```python
from build123d import *

# Parameters (mm, degrees)
F0_R     = 2.1
F1_DEPTH = 2
F2_R     = 4.1
F2_R_2   = 2.1
F3_DEPTH = 2.67
F4_W     = 1
F4_H     = 4.975
F4_W_2   = 3.1
F5_DEPTH = 5


with BuildPart() as f1:
    # F0 (on Top) → F1 (new body)
    with BuildSketch(Plane.XY):
        with BuildLine():
            Line((0, 15), (0, 0))
            Line((0, 0), (17, 0))
            ThreePointArc((17, 0), (24.5, 7.5), (17, 15))
            Line((17, 15), (0, 15))
        make_face()
        with Locations((17, 7.5)):
            Circle(F0_R, mode=Mode.SUBTRACT)
    extrude(amount=F1_DEPTH)

    # F2 (on face) → F3 (join)
    with BuildSketch(Plane.XY.offset(2)):
        with Locations((17, 7.5)):
            Circle(F2_R)
        with Locations((17, 7.5)):
            Circle(F2_R_2, mode=Mode.SUBTRACT)
    extrude(amount=F3_DEPTH)

    # F4 (on face) → F5 (join)
    with BuildSketch(Plane(origin=(0, 0, 0), x_dir=(1, 0, 0), z_dir=(0, 0, -1))):
        with Locations((3.3, -3.9125)):
            Rectangle(F4_W, F4_H)
        with Locations((7.45, -3.9125)):
            Rectangle(F4_W_2, F4_H)
        with BuildLine():
            ThreePointArc((22.529693, -6.05), (22.771721, -5.927264), (22.815711, -5.659483))
            ThreePointArc((22.815711, -5.659483), (21.102936, -2.986031), (18.278593, -1.535505))
            ThreePointArc((18.278593, -1.535505), (18.027117, -1.595534), (17.915711, -1.828841))
            Line((17.915711, -1.828841), (17.915711, -3.503567))
            ThreePointArc((17.915711, -3.503567), (19.695084, -4.410256), (20.835036, -6.05))
            Line((20.835036, -6.05), (22.529693, -6.05))
        make_face()
        with BuildLine():
            ThreePointArc((17.915711, -13.171159), (18.027117, -13.404466), (18.278593, -13.464495))
            ThreePointArc((18.278593, -13.464495), (21.102936, -12.013969), (22.815711, -9.340517))
            ThreePointArc((22.815711, -9.340517), (22.771721, -9.072736), (22.529693, -8.95))
            Line((22.529693, -8.95), (20.835036, -8.95))
            ThreePointArc((20.835036, -8.95), (19.695084, -10.589744), (17.915711, -11.496433))
            Line((17.915711, -11.496433), (17.915711, -13.171159))
        make_face()
        with Locations((3.3, -11.0875)):
            Rectangle(F4_W, F4_H)
        with Locations((7.45, -11.0875)):
            Rectangle(F4_W_2, F4_H)
    extrude(amount=F5_DEPTH)


solid = f1.part
```
Design review of the part built by this model. Coordinates are the model's own, in mm. A direction names the side the tool comes from. Give positions to 0.01 mm unless a question says otherwise; leave off trailing zeros. Loops run counter-clockwise (first coordinate to the right, second up) from the corner with the lowest first, then second, coordinate; pieces in that order, holes last. Notation, with made-up numbers: M 42,88.5 L 54,88.5 A16 cw 54,115.5 Z; hole C -34.5,59.5 d4. An arc over 180 degrees is marked long. Return JSON: item names as keys, results as strings. Group by question number.
Item 1: Tool access review of faces 1 (the flat face through (7, 8.6, -2)), 2 (the flat face through (5.9, 11, -2)), 3 (the flat face through (3, 1.425, -2)), 4 (the cylindrical face through (12.904, 7.68, 3.316)), 5 (the flat face through (22, 8.95, -2)): name each direction out of +Z, -Z, +X, -X, +Y, -Y from which nothing blocks a thin tool from reaching the whole face with its end or side.
Item 2: We need section A-A (z = -3.5). Give the number of separate pieces and of enclosed holes in the cut face, and give its area (3 significant figures).
Item 3: Mouldability with a two-part tool opening along X and no side actions: class faces 6 (the flat face through (3.8, 11, -2)), 7 (the flat face through (7, 13.575, -2)), 8 (the cylindrical face through (21.07, 12.044, -2.465)), 9 (the cylindrical face through (16.727, 9.582, 2.302)) as released by +X, released by -X, zero draft, split by the parting line, or undercut.
Item 4: We need section D-D (z = 1.75). Give the boundary of the cut face in (x, y).
Item 5: For probe 1 along Y at (x, z) = (17, 3); probe 2 along Y at (x, z) = (3.75, -2) (3 decimals); probe 3 along X at (y, z) = (10.75, -0.25), list the stretches that pass through material, from the lowest coordinate up.
Item 6: We need section B-B (y = 7.5). Give the boundary of the cut face in (x, z).
Item 7: We need section C-C (x = 7). Give the boundary of the cut face in (y, z) (3 decimals), and give its area (4 significant figures).
Item 8: Insertion check: pin 1 Ø4 at (y, z) = (9, -1) entering from -X; pin 2 Ø1.5 at (y, z) = (4, -2) entering from -X; pin 3 Ø1.5 at (y, z) = (7.5, -2.5) entering from -X; pin 4 Ø1.5 at (y, z) = (4, -1.5) entering from +X. Each pin has a flat end and moves straight along its axis. Give the tip position at first contact, or say it passes through.
Output:
{
 "1": {"face 1": "-Z, +X, -X", "face 2": "-Z, +Y, -Y", "face 3": "-Z, +X, -X, -Y", "face 4": "+Z", "face 5": "-Z, +X"},
 "2": {"separate pieces": "6", "enclosed holes": "0", "area": "63.1 mm^2"},
 "3": {"face 6": "undercut", "face 7": "zero draft", "face 8": "released by +X", "face 9": "undercut"},
 "4": {"outline": "M 0,0 L 17,0 A7.5 ccw 17,15 L 0,15 Z; hole C 17,7.5 d4.2"},
 "5": {"probe 1": "y = 3.4 to 5.4, 9.6 to 11.6", "probe 2": "y = 1.425 to 6.4, 8.6 to 13.575", "probe 3": "x = 2.8 to 3.8, 5.9 to 9, 19.5 to 22.16"},
 "6": {"outline": "M 0,0 L 14.9,0 L 14.9,4.67 L 12.9,4.67 L 12.9,2 L 0,2 Z; M 19.1,0 L 24.5,0 L 24.5,2 L 21.1,2 L 21.1,4.67 L 19.1,4.67 Z"},
 "7": {"outline": "M 0,0 L 1.425,0 L 1.425,-5 L 6.4,-5 L 6.4,0 L 8.6,0 L 8.6,-5 L 13.575,-5 L 13.575,0 L 15,0 L 15,2 L 0,2 Z", "area": "79.75 mm^2"},
 "8": {"pin 1": "stops at x = 0", "pin 2": "stops at x = 2.8", "pin 3": "passes through", "pin 4": "stops at x = 22.44"}
}
